Input: part model. Units: mm. Frame: model coordinates. A direction names the side the tool comes from. Coordinates: 2 decimals unless noted, no trailing zeros. Order: outer loops, then holes, each group sorted by start corner. A loop starts at its lowest first (then second) coordinate and runs counter-clockwise, first axis right, second up. Notation, with made-up numbers: M 57.25,34 L 108.25,34 A17 ccw 108.25,56 Z; hole C 57,35.25 d11. An arc over 180 degrees is marked long. Answer in a Markdown table with one row per item.
from build123d import *

# Parameters (mm, degrees)
F0_W      = 69
F0_H      = 27
F1_DEPTH  = 2
F2_W      = 40
F2_H      = 30
F3_DEPTH  = 5.6
F4_W      = 35
F4_H      = 18
F5_DEPTH  = 5
F6_W      = 15
F6_H      = 12
F7_DEPTH  = 5
F8_R      = 5.5
F9_DEPTH  = 8.5
F11_DEPTH = 4


with BuildPart() as f1:
    # F0 (on Front) → F1 (new body)
    with BuildSketch(Plane.XZ):
        Rectangle(F0_W, F0_H)
    extrude(amount=F1_DEPTH)

    # F2 (on face) → F3 (join)
    with BuildSketch(Plane.XZ.offset(2)):
        with Locations((-40.5, 0)):
            Rectangle(F2_W, F2_H)
    extrude(amount=F3_DEPTH)

    # F4 (on face) → F5 (join)
    with BuildSketch(Plane.XZ.offset(2)):
        Rectangle(F4_W, F4_H)
    extrude(amount=F5_DEPTH)

    # F6 (on face) → F7 (join)
    with BuildSketch(Plane.XZ.offset(2)):
        with Locations((25, 5.5)):
            Rectangle(F6_W, F6_H)
    extrude(amount=F7_DEPTH)

    # F8 (on face) → F9 (join)
    with BuildSketch(Plane.XZ.offset(2)):
        with Locations((26.5, -8)):
            Circle(F8_R)
    extrude(amount=F9_DEPTH)

    # F10 (on face) → F11 (join)
    with BuildSketch(Plane.XZ.offset(7.6)):
        with BuildLine():
            Line((-35.5, 12.5), (-52.5, 12.5))
            ThreePointArc((-52.5, 12.5), (-54.62132, 11.62132), (-55.5, 9.5))
            Line((-55.5, 9.5), (-55.5, -9.5))
            ThreePointArc((-55.5, -9.5), (-54.62132, -11.62132), (-52.5, -12.5))
            Line((-52.5, -12.5), (-35.5, -12.5))
            ThreePointArc((-35.5, -12.5), (-33.37868, -11.62132), (-32.5, -9.5))
            Line((-32.5, -9.5), (-32.5, 9.5))
            ThreePointArc((-32.5, 9.5), (-33.37868, 11.62132), (-35.5, 12.5))
        make_face()
    extrude(amount=F11_DEPTH)


solid = f1.part
1) Mould query, pull axis X, two halves, no side actions, for faces 1 (the face through (-33.4, -9.57, -11.64)), 2 (the face through (-45, -2, 0)), 3 (the face through (-33.36, -9.57, 11.6)). Classes: +X half, -X half, draft (parallel to the pull), parting line (faces both ways), or undercut.
Resolved:
| item | result |
|---|---|
| face 1 | undercut |
| face 2 | draft |
| face 3 | +X half |
2) Cut plane A-A, the plane x = -8.5. Output: boundary loops of the cut face in (y, z).
Resolved:
| item | result |
|---|---|
| outline | M -7,-9 L -2,-9 L -2,-13.5 L 0,-13.5 L 0,13.5 L -2,13.5 L -2,9 L -7,9 Z |
3) Reachability of faces 4 (the face through (25, -4, -0.5)), 5 (the face through (17.5, -4, 10)), 6 (the face through (-44, -10, 12.5)), 7 (the face through (0, -4, -9)), 8 (the face through (-44, -10, -12.5)) from +Z, -Z, +X, -X, +Y, -Y: full face, straight path, thin tool, end or side. Return the list, or none.
Resolved:
| item | result |
|---|---|
| face 4 | +X, -Y |
| face 5 | +Z, -Y |
| face 6 | +Z, +X, -X, -Y |
| face 7 | -Z, -Y |
| face 8 | -Z, -X, -Y |
4) Material intervals for probe 1 along X at (y, z) = (-6, -8.5); probe 2 along X at (y, z) = (-5.5, 10.5); probe 3 along X at (y, z) = (-3.75, 4.25), sorted ascending.
Resolved:
| item | result |
|---|---|
| probe 1 | x = -60.5 to -20.5, -17.5 to 17.5, 21.02 to 31.98 |
| probe 2 | x = -60.5 to -20.5, 17.5 to 32.5 |
| probe 3 | x = -60.5 to -20.5, -17.5 to 32.5 |
5) Contact query for flat-ended pins moving along their axis: pin 1 (12 mm diameter, centred on x = -46.5, z = 11, fed in from +Y); pin 2 (6 mm diameter, centred on x = 18, y = -5.5, fed in from -Z); pin 3 (5.5 mm diameter, centred on x = 26, z = -10.5, fed in from -Y). Output: stop coordinate, or through.
Resolved:
| item | result |
|---|---|
| pin 1 | stops at y = -2 |
| pin 2 | stops at z = -9 |
| pin 3 | stops at y = -10.5 |
6) Cut plane C-C, the plane z = 2.25. Output: boundary loops of the cut face in (x, y).
Resolved:
| item | result |
|---|---|
| outline | M -60.5,-7.6 L -55.5,-7.6 L -55.5,-11.6 L -32.5,-11.6 L -32.5,-7.6 L -20.5,-7.6 L -20.5,-2 L -17.5,-2 L -17.5,-7 L 32.5,-7 L 32.5,-2 L 34.5,-2 L 34.5,0 L -34.5,0 L -34.5,-2 L -60.5,-2 Z |
7) Cut plane B-B, the plane z = -8. Output: boundary loops of the cut face in (x, y).
Resolved:
| item | result |
|---|---|
| outline | M -60.5,-7.6 L -55.5,-7.6 L -55.5,-11.6 L -32.5,-11.6 L -32.5,-7.6 L -20.5,-7.6 L -20.5,-2 L -17.5,-2 L -17.5,-7 L 17.5,-7 L 17.5,-2 L 21,-2 L 21,-10.5 L 32,-10.5 L 32,-2 L 34.5,-2 L 34.5,0 L -34.5,0 L -34.5,-2 L -60.5,-2 Z |
